CAD build for the part. Positions are in the model's coordinates, mm. Give positions to 0.01 mm unless a question says otherwise; leave off trailing zeros. Loops run counter-clockwise (first coordinate to the right, second up) from the corner with the lowest first, then second, coordinate; pieces in that order, holes last.
Item 1: Saw through at B-B on z = 2.5. Give the number of separate pieces and of enclosed holes in the cut face, plus the area to 3 significant figures.
Item 2: Probe probe 1 along X at (y, z) = (-62.5, 1.75); probe 2 along X at (y, z) = (-64, 6); probe 3 along Y at (x, z) = (-85, 5). List the from-to ranges inside material, lowest first.
Item 3: Saw through at A-A on x = 80. Give the cut face in (y, z), plus the area to 3 significant figures.
Item 4: Drop a flat-ended pin along its axis: P1, Ø5, axis at y = -76.5, z = 5.5, coming from the +X side. Give the stop position or say it passes through.
Item 5: Saw through at C-C on x = -75. Give the cut face in (y, z), plus the area to 3 significant figures.
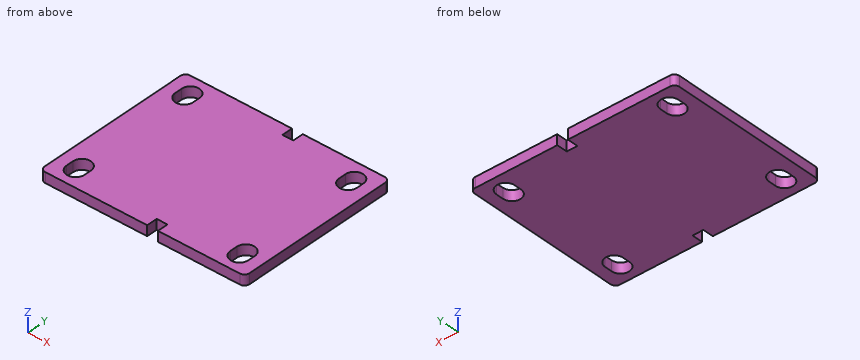
from build123d import *

# Parameters (mm, degrees)
ESQUISSE1_W             = 200
ESQUISSE1_H             = 160
ESQUISSE1_R             = 8.75
BOSS_EXTRU_1_DEPTH      = 10
ESQUISSE2_W             = 10.5
ESQUISSE2_H             = 10.5
ENL_V_MAT_EXTRU_1_DEPTH = 10
CONG_1_R                = 5
ENL_V_MAT_EXTRU_2_DEPTH = 11
SYM_TRIE2_COPY_1_DEPTH  = 11


with BuildPart() as part:
    # Esquisse1 → Boss.-Extru.1 (new body)
    with BuildSketch(Plane.XY):
        Rectangle(ESQUISSE1_W, ESQUISSE1_H)
        with Locations((-80, 60)):
            Circle(ESQUISSE1_R, mode=Mode.SUBTRACT)
        with Locations((80, 60)):
            Circle(ESQUISSE1_R, mode=Mode.SUBTRACT)
        with Locations((80, -60)):
            Circle(ESQUISSE1_R, mode=Mode.SUBTRACT)
        with Locations((-80, -60)):
            Circle(ESQUISSE1_R, mode=Mode.SUBTRACT)
    extrude(amount=BOSS_EXTRU_1_DEPTH)

    # Esquisse2 → Enlèv. mat.-Extru.1 (cut)
    with BuildSketch(Plane.XY.offset(10)):
        with Locations((9.75, 74.75)):
            Rectangle(ESQUISSE2_W, ESQUISSE2_H)
        with Locations((9.75, -74.75)):
            Rectangle(ESQUISSE2_W, ESQUISSE2_H)
    extrude(amount=-ENL_V_MAT_EXTRU_1_DEPTH, mode=Mode.SUBTRACT)

    # Congé1
    cong_1_edges = [part.edges().sort_by_distance(p)[0] for p in [
        (-100, 80, 5),
        (100, 80, 5),
        (100, -80, 5),
        (-100, -80, 5),
    ]]
    fillet(cong_1_edges, radius=CONG_1_R)

    # Esquisse3 → Enlèv. mat.-Extru.2 (cut, through all)
    with BuildSketch(Plane.XY.offset(10)):
        with BuildLine():
            Line((-71.25, 63.5), (-71.25, 56.5))
            ThreePointArc((-71.25, 56.5), (-80, 47.75), (-88.75, 56.5))
            Line((-88.75, 56.5), (-88.75, 63.5))
            ThreePointArc((-88.75, 63.5), (-80, 72.25), (-71.25, 63.5))
        make_face()
    enl_v_mat_extru_2 = extrude(amount=-ENL_V_MAT_EXTRU_2_DEPTH, mode=Mode.SUBTRACT)

    # Symétrie1: Enlèv. mat.-Extru.2 across plane
    add(enl_v_mat_extru_2.mirror(Plane.ZX), mode=Mode.SUBTRACT)

    # Symétrie2: Enlèv. mat.-Extru.2 across plane
    add(enl_v_mat_extru_2.mirror(Plane(origin=(0, 0, 0), x_dir=(0, 0, 1), z_dir=(1, 0, 0))), mode=Mode.SUBTRACT)

    # Symétrie2 copy 1 sketch → Symétrie2 copy 1 (cut, through all)
    with BuildSketch(Plane(origin=(0, 0, 10), x_dir=(-1, 0, 0), z_dir=(0, 0, 1))):
        with BuildLine():
            Line((-71.25, 63.5), (-71.25, 56.5))
            ThreePointArc((-71.25, 56.5), (-80, 47.75), (-88.75, 56.5))
            Line((-88.75, 56.5), (-88.75, 63.5))
            ThreePointArc((-88.75, 63.5), (-80, 72.25), (-71.25, 63.5))
        make_face()
    extrude(amount=-SYM_TRIE2_COPY_1_DEPTH, mode=Mode.SUBTRACT)


solid = part.part
Results below:
1. separate pieces: 1
1. enclosed holes: 4
1. area: 30,300 mm2
2. probe 1: x = -100 to -88.75, -71.25 to 71.25, 88.75 to 100
2. probe 2: x = -100 to -88.74, -71.26 to 71.26, 88.74 to 100
2. probe 3: y = -80 to -70.68, -49.32 to 49.32, 70.68 to 80
3. outline: (-80, 0) - (-72.25, 0) - (-72.25, 10) - (-80, 10) - close; (-47.75, 0) - (47.75, 0) - (47.75, 10) - (-47.75, 10) - close; (72.25, 0) - (80, 0) - (80, 10) - (72.25, 10) - close
3. area: 1,110 mm2
4. P1: stops at x = 100
5. outline: (-80, 0) - (-70.68, 0) - (-70.68, 10) - (-80, 10) - close; (-49.32, 0) - (49.32, 0) - (49.32, 10) - (-49.32, 10) - close; (70.68, 0) - (80, 0) - (80, 10) - (70.68, 10) - close
5. area: 1,170 mm2
